Can you work these out from the drawing? Everything is in mm from the part's minimum corner. A direction names the side the tool comes from. Round coordinates to 2 decimals unless told otherwise and drop trailing zeros. Loops run counter-clockwise (first coordinate to the right, second up) from the corner with the lowest first, then second, coordinate; pieces in that order, holes last. Notation, with made-up numbers: (52, 10.5) - (79, 10.5) arc R15 ccw to (79, 15.5) - close; hole circle Ø7 at (-2, 0). An arc over 180 degrees is marked (long way). Answer as a JSON object with one key per item and string values. Group by question number.
1) I want a section at B-B, the plane y = 10. Please give me the cut outline in (x, z).
2) I want a section at A-A, the plane z = 14. Please give me the cut outline in (x, y), then the cut area to 3 significant figures.
3) If I drill on line 1 along Y through (x, z) = (10.5, 24.25); line 2 along X through (y, z) = (31.5, 4.5); line 3 along X through (y, z) = (39.5, 12.5), over which ranges is the centre line in solid material (lowest first)? Write a range as [from, to].
4) Which directions (+Z, -Z, +X, -X, +Y, -Y) give clear straight access to the entire face, cutting with the end or side of a thin tool? Please do the marked faces 3 and 4.
5) Will these pins go through, and if not, where does the flat tip stop? P1, Ø2, axis at x = 20.5, y = 31.5, coming from the -Z side; P2, Ø1.5, axis at x = 4, y = 29, coming from the -Z side; P3, Ø3, axis at y = 10, z = 24.5, coming from the -X side.
6) If we mould it in two halves opening along X, with no side actions, what happens to the marked faces 1 and 2? For each: pulls with the +X half, pulls with the -X half, needs draft (parallel to the pull), parting line crosses it, or undercut.
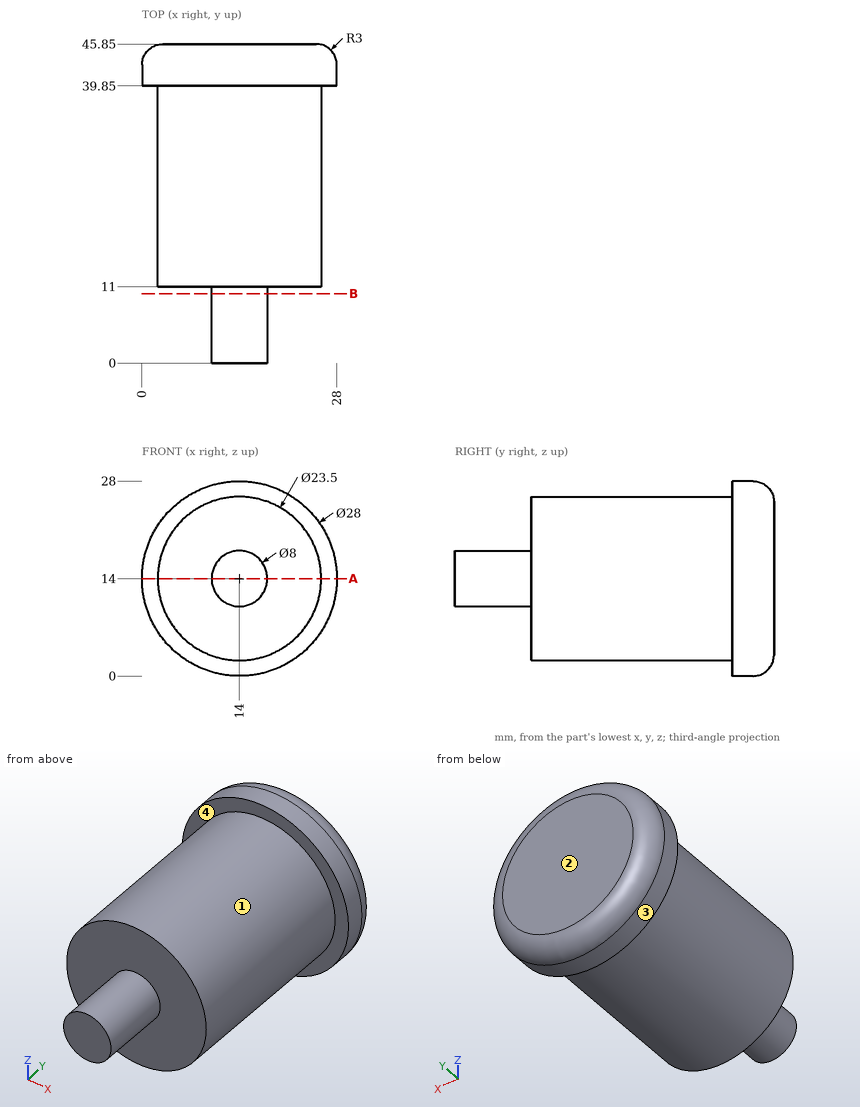
Outcome:
{
 "1": {"outline": "circle Ø8 at (14, 14)"},
 "2": {"outline": "(0, 39.85) - (2.25, 39.85) - (2.25, 11) - (10, 11) - (10, 0) - (18, 0) - (18, 11) - (25.75, 11) - (25.75, 39.85) - (28, 39.85) - (28, 42.85) arc R3 ccw to (25, 45.85) - (3, 45.85) arc R3 ccw to (0, 42.85) - close", "area": "930 mm^2"},
 "3": {"line 1": "[11, 45.85]", "line 2": "[7.09, 20.91]", "line 3": "[2.35, 25.65]"},
 "4": {"face 3": "+Y, -Y", "face 4": "-Y"},
 "5": {"P1": "z = 3.62", "P2": "z = 6.75", "P3": "x = 6.93"},
 "6": {"face 1": "parting line crosses it", "face 2": "needs draft"}
}
